The drawing under review shows one solid part. Ordinate dimensions are in mm from its lowest x, y, z. A direction names the side the tool comes from. Give positions to 0.01 mm unless a question says otherwise; leave off trailing zeros. Write each loop counter-clockwise with the first axis right and the second up, starting at its lowest first coordinate (ties: lowest second). Pieces come first, ordered by that corner, then holes.
Q1. Machinability: for the marked faces 1, 2 and 3, which of the approach directions +Z, -Z, +X, -X, +Y, -Y give a long, thin tool a straight path to every point of the face, cutting with its end or side? Answer none if there is none.
Q2. We need section A-A (y = 9). Write out the cut boundary in (x, z).
Q3. We need section C-C (z = 1.6). Write out the cut boundary in (x, y), then the cut area to 3 significant figures.
Q4. For line 1 (Y direction, x = 9, z = 0.7); line 2 (Y direction, x = 9, z = 2.2), list the stretches that pass through material, from the lowest coordinate up.
Q5. Mouldability with a two-part tool opening along X and no side actions: class the marked faces 4, 5 and 6 as released by +X, released by -X, zero draft, split by the parting line, or undercut.
Q6. Insertion check: P1, Ø1.2, axis at x = 8.5, y = 9, coming from the +Z side; P2, Ø1.5, axis at x = 4.5, z = 2.5, coming from the +Y side; P3, Ø3.5, axis at x = 9, y = 9, coming from the -Z side. Each pin has a flat end and moves straight along its axis. Give the tip position at first contact, or say it passes through.
Q7. We need section D-D (x = 16.25). Write out the cut boundary in (y, z).
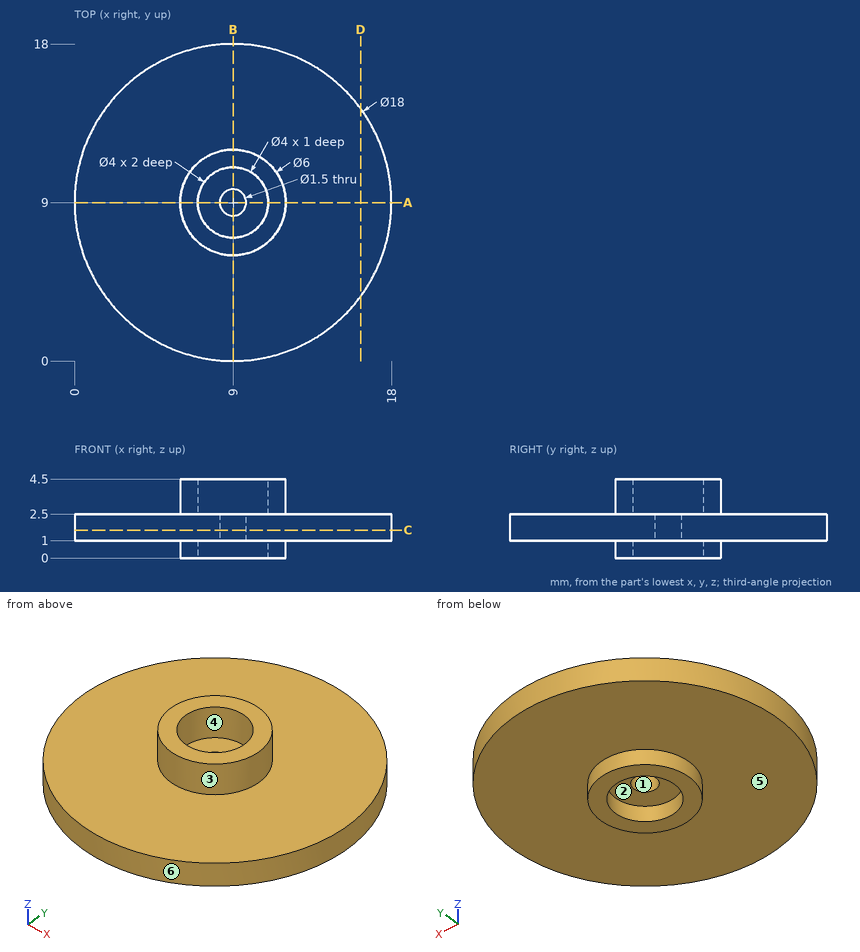
Computed:
1. face 1: +Z, -Z
1. face 2: -Z
1. face 3: +Z
2. outline: (0, 1) - (6, 1) - (6, 0) - (7, 0) - (7, 1) - (8.25, 1) - (8.25, 2.5) - (7, 2.5) - (7, 4.5) - (6, 4.5) - (6, 2.5) - (0, 2.5) - close; (9.75, 1) - (11, 1) - (11, 0) - (12, 0) - (12, 1) - (18, 1) - (18, 2.5) - (12, 2.5) - (12, 4.5) - (11, 4.5) - (11, 2.5) - (9.75, 2.5) - close
3. outline: circle Ø18 at (9, 9); hole circle Ø1.5 at (9, 9)
3. area: 253 mm2
4. line 1: y = 6 to 7, 11 to 12
4. line 2: y = 0 to 8.25, 9.75 to 18
5. face 4: undercut
5. face 5: zero draft
5. face 6: split by the parting line
6. P1: stops at z = 2.5
6. P2: stops at y = 17.18
6. P3: stops at z = 1
7. outline: (3.67, 1) - (14.33, 1) - (14.33, 2.5) - (3.67, 2.5) - close
